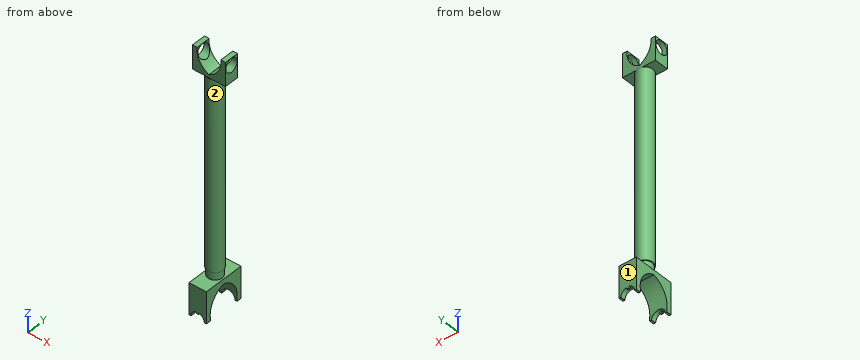
Autodesk Inventor part; units mm, degrees
ref_plane "YZ Plane" through (0, 0, 0) normal (1, 0, 0) x (0, 1, 0)
ref_plane "XZ Plane" through (0, 0, 0) normal (0, 1, 0) x (-1, 0, 0)
ref_plane "XY Plane" through (0, 0, 0) normal (0, 0, 1) x (1, 0, 0)
sketch "Sketch1" plane through (0, 0, 0) normal (0, 0, 1) x (1, 0, 0)
  circle A0 centre (0, 0) radius 5
  dimension "d0" = 10
extrude "Extrusion1" add sketch "Sketch1" against normal blind 120
sketch "Sketch2" plane through (0, 0, -120) normal (0, 0, -1) x (-1, 0, 0)
  circle A0 centre (0, 0) radius 4.5
  dimension "d3" = 9
extrude "Extrusion2" add sketch "Sketch2" along normal blind 5
sketch "Sketch3" plane through (0, 0, 0) normal (0, 0, 1) x (1, 0, 0)
  circle A0 centre (0, 0) radius 5
  line L0 (0, 0) -> (10, 0)
  line L1 (10, 0) -> (-10.5, 0)
  line L2 (0, 0) -> (0, 4.5)
  line L3 (0, 4.5) -> (0, -4.5)
  line L4 (0, -4.5) -> (-10.5, -4.5)
  line L5 (-10.5, -4.5) -> (-10.5, 0)
  line L6 (-10.5, 0) -> (-10.5, 4.5)
  line L7 (-10.5, 4.5) -> (0, 4.5)
  line L8 (0, 4.5) -> (10.5, 4.5)
  line L9 (10.5, 4.5) -> (10.5, -4.5)
  line L10 (10.5, -4.5) -> (0, -4.5)
  dimension "d8" = 4.5
  dimension "d50" = 10.5
  dimension "d52" = 10.5
  dimension "d53" = 4.5
extrude "Extrusion3" add sketch "Sketch3" along normal blind 15 contours L0 L2 L8 A0 | A0 L8 L9 L10 | A0 L10 L3 L0 | L3 L4 A0 L1 | L1 A0 L7 L2 | A0 L1 L6 L7 | L4 L5 L1 A0
sketch "Sketch4" plane through (-10.5, -4.5, 0) normal (0, -1, 0) x (1, 0, 0)
  line L0 (0, 0) -> (8.3206, 0)
  line L1 (12.6794, 0) -> (8.3206, 0)
  line L2 (12.6794, 0) -> (21, 0)
  line L3 (21, 0) -> (21, 15)
  line L4 (0, 15) -> (21, 15)
  line L5 (0, 0) -> (0, 15)
  line L6 (10.5, 0) -> (10.5, 2)
  line L7 (0, 15) -> (21, 15)
  line L8 (0, 15) -> (3, 15)
  line L9 (21, 15) -> (18, 15)
  arc A0 (3, 15) -> (10.5, 2) centre (15.2653, 13.4127) ccw
  line L10 (10.5, 2) -> (10.5, 15)
  line L11 (4.5527, 7.2323) -> (0, 7.2323)
  line L12 (0, 0) -> (0, 15)
  line L13 (4.5527, 7.2323) -> (4.5527, 0)
  line L14 (16.4473, 7.2323) -> (21, 7.2323)
  line L15 (16.4473, 7.2323) -> (16.4473, 0)
  arc A1 (10.5, 2) -> (18, 15) centre (5.7347, 13.4127) ccw
  dimension "d12" = 2
  dimension "d13" = 3
  dimension "d14" = 3
extrude "Extrusion4" cut sketch "Sketch4" against normal blind 15 contours A0 L4 L10 | L10 L4 A1
sketch "Sketch5" plane through (10.5, -4.5, 0) normal (1, 0, 0) x (0, 0, -1)
  line L0 (0, 0) -> (0, 9)
  line L1 (0, 9) -> (-15, 9)
  line L2 (-15, 0) -> (-15, 9)
  line L3 (0, 0) -> (-15, 0)
  line L4 (-15, 0) -> (-15, 9)
  line L5 (-15, 4.5) -> (-10.5, 4.5)
  line L6 (0, 9) -> (0, 0)
  circle A0 centre (-10.5, 4.5) radius 4.25
  point P0 (0, 4.5)
  dimension "d19" = 4.5
  dimension "d20" = 8.5
extrude "Extrusion5" cut sketch "Sketch5" against normal blind 37.25 contours A0
sketch "Sketch6" plane through (0, 0, -125) normal (0, 0, -1) x (-1, 0, 0)
  circle A0 centre (0, 0) radius 4.5
  line L0 (0, 0) -> (0, 13)
  line L1 (0, -4.5) -> (0, 4.5)
  line L2 (0, 13) -> (0, -13)
  line L3 (0, -13) -> (-5.5, -13)
  line L4 (-5.5, -13) -> (5.5, -13)
  line L5 (5.5, -13) -> (5.5, 13)
  line L6 (5.5, 13) -> (-5.5, 13)
  line L7 (-5.5, 13) -> (-5.5, -13)
  dimension "d23" = 13
  dimension "d24" = 26
  dimension "d25" = 5.5
  dimension "d26" = 11
extrude "Extrusion6" add sketch "Sketch6" along normal blind 25
sketch "Sketch7" plane through (5.5, -13, -125) normal (1, 0, 0) x (0, 0, -1)
  line L0 (0, 26) -> (0, 0)
  line L1 (0, 0) -> (25, 0)
  line L2 (25, 26) -> (25, 0)
  line L3 (0, 26) -> (25, 26)
  line L4 (25, 26) -> (25, 0)
  line L5 (25, 26) -> (25, 23)
  line L6 (25, 0) -> (25, 3)
  line L7 (25, 23) -> (18, 23)
  line L8 (0, 8.5) -> (0, 17.5)
  line L9 (0, 13) -> (3, 13)
  arc A0 (18, 23) -> (3, 13) centre (16.2622, 9.3566) ccw
  line L10 (25, 3) -> (18, 3)
  line L11 (18, 3) -> (18, 23)
  arc A1 (3, 13) -> (18, 3) centre (16.3321, 16.7481) ccw
  point P0 (-125, 13)
  dimension "d29" = 3
  dimension "d30" = 3
  dimension "d32" = 7
  dimension "d33" = 3
extrude "Extrusion7" cut sketch "Sketch7" against normal blind 25 contours L2 L10 L11 L7 | A0 L11 A1
sketch "Sketch8" plane through (-5.5, 13, -125) normal (0, 1, 0) x (1, 0, 0)
  line L0 (0, 0) -> (11, 0)
  line L1 (11, 0) -> (11, 25)
  line L2 (0, 25) -> (11, 25)
  line L3 (0, 0) -> (0, 25)
  line L4 (5.5, 25) -> (5.5, 20)
  circle A0 centre (5.5, 20) radius 4.25
  line L5 (1.25, 20) -> (0, 20)
  line L6 (0, 18) -> (0, 25)
  line L7 (9.75, 20) -> (11, 20)
  line L8 (11, 25) -> (11, 18)
  point P0 (5.5, -125)
  dimension "d36" = 5
  dimension "d37" = 8.5
extrude "Extrusion8" cut sketch "Sketch8" against normal blind 30 contours L3 L2 L4 A0 L5 | L7 A0 L4 L2 L1 | A0
sketch "Sketch9" plane through (-5.5, 13, -125) normal (0, 1, 0) x (1, 0, 0)
  line L0 (1.25, 20) -> (0, 20)
  line L1 (0, 0) -> (0, 20)
  line L2 (0, 0) -> (11, 0)
  line L3 (11, 0) -> (11, 20)
  line L4 (11, 20) -> (9.75, 20)
  arc A0 (1.25, 20) -> (9.75, 20) centre (5.5, 20) ccw
  arc A1 (1.25, 20) -> (9.75, 20) centre (5.5, 20) ccw
  line L5 (5.5, 15.75) -> (5, 15.75)
  line L6 (5, 15.75) -> (4.5, 15.75)
  line L7 (4.5, 15.75) -> (6.5, 15.75)
  line L8 (6.5, 15.75) -> (6.1213, 16.7351)
  line L9 (6.1213, 16.7351) -> (5.5, 16.7351)
  line L10 (5.5, 16.7351) -> (5.5, 15.75)
  line L11 (4.5, 15.75) -> (4.8787, 16.7351)
  line L12 (4.8787, 16.7351) -> (5.5, 16.7351)
  line L13 (0, 20) -> (1.25, 20)
  arc A2 (1.25, 20) -> (9.75, 20) centre (5.5, 20) ccw
  line L14 (9.75, 20) -> (11, 20)
  line L15 (11, 0) -> (11, 20)
  line L16 (11, 0) -> (0, 0)
  line L17 (0, 0) -> (0, 20)
  point P0 (5.5, -125)
  point P1 (4.5421, 15.8594)
  point P2 (6.4579, 15.8594)
  dimension "d40" = 0.5
  dimension "d41" = 0.5
  dimension "d42" = 2
extrude "Extrusion9" add sketch "Sketch9" against normal blind 1 contours L11 L12 L10 A0 | L10 L9 L8 A0
sketch "Sketch10" plane through (-5.5, -13, -125) normal (0, -1, 0) x (1, 0, 0)
  line L0 (0, -20) -> (1.25, -20)
  arc A0 (9.75, -20) -> (1.25, -20) centre (5.5, -20) ccw
  line L1 (9.75, -20) -> (11, -20)
  line L2 (11, 0) -> (11, -20)
  line L3 (11, 0) -> (0, 0)
  line L4 (0, 0) -> (0, -20)
  arc A1 (6.4579, -15.8594) -> (4.5421, -15.8594) centre (5.5, -20) ccw
  line L5 (5.5, -15.75) -> (4.5, -15.75)
  line L6 (4.5, -15.75) -> (6.5, -15.75)
  line L7 (6.1213, -16.7351) -> (6.4579, -15.8594)
  line L8 (6.5, -15.75) -> (6.1213, -16.7351)
  line L9 (4.5421, -15.8594) -> (4.8787, -16.7351)
  line L10 (6.1213, -16.7351) -> (4.8787, -16.7351)
  line L11 (4.8787, -16.7351) -> (4.5, -15.75)
  point P0 (5.5, 125)
  dimension "d45" = 1
  dimension "d46" = 2
extrude "Extrusion10" add sketch "Sketch10" against normal blind 1 contours A0 L7 L10 L9
Source: CAD feature listing. Evaluate the final solid. Frame: model axes, mm. Face numbers are marked on the shaded views. Coordinates: 2 decimals unless noted, no trailing zeros. Loops run counter-clockwise (first coordinate to the right, second up) from the corner with the lowest first, then second, coordinate; pieces in that order, holes last. Notation, with made-up numbers: (2, -21) -> (59, -21) arc R21 ccw to (59, 5) -> close; hole circle Ø3 at (70.5, 25). An arc over 180 degrees is marked (long way). Answer in a Markdown table with one row per item. Add a question column.
Q1. Contact query for flat-ended pins moving along their axis: pin 1 Ø8 at (x, z) = (-1, -33.5) entering from -Y; pin 2 Ø7.5 at (y, z) = (0, 10.5) entering from -X; pin 3 Ø5 at (y, z) = (0.5, -64) entering from -X; pin 4 Ø0.8 at (x, y) = (0.5, 12.5) entering from -Z. Output: stop coordinate, or through.
Q2. Section C-C on z = -37.5. Return the cut outline in (x, y), and give its area (3 significant figures).
Q3. Ray query, line 1 along Y through (x, z) = (8.9, 10.5); line 2 along Z through (x, y) = (8.95, 0); line 3 along X through (y, z) = (-2.5, -121.5). Return the intervals inside material, ascending.
Q4. Section B-B on y = -2.75. Return the cut outline in (x, z).
Q5. Pull-direction query (Z, two-part tool) for the marked faces 1 and 2; classes: pulls with the +Z half, pulls with the -Z half, needs draft (parallel to the pull), parting line crosses it, or undercut.
Q6. Section A-A on z = 10.5. Return the cut outline in (x, y).
Computed values:
| question | item | result |
|---|---|---|
| 1 | pin 1 | stops at y = -5 |
| 1 | pin 2 | passes through |
| 1 | pin 3 | stops at x = -5 |
| 1 | pin 4 | stops at z = -141.74 |
| 2 | outline | circle Ø10 at (0, 0) |
| 2 | area | 78.5 mm^2 |
| 3 | line 1 | y = -4.5 to -4.25, 4.25 to 4.5 |
| 3 | line 2 | z = 0 to 6.25, 14.75 to 15 |
| 3 | line 3 | x = -3.74 to 3.74 |
| 4 | outline | (-10.5, 0) -> (-4.18, 0) -> (-4.18, -120) -> (-3.56, -120) -> (-3.56, -125) -> (-5.5, -125) -> (-5.5, -129.1) -> (5.5, -129.1) -> (5.5, -125) -> (3.56, -125) -> (3.56, -120) -> (4.18, -120) -> (4.18, 0) -> (10.5, 0) -> (10.5, 7.26) -> (5.96, 7.26) arc R12.37 cw to (0, 2) arc R12.37 cw to (-5.96, 7.26) -> (-10.5, 7.26) -> close; (-10.5, 13.74) -> (-7.6, 13.74) arc R12.37 cw to (-7.5, 15) -> (-10.5, 15) -> close; (7.5, 15) arc R12.37 cw to (7.6, 13.74) -> (10.5, 13.74) -> (10.5, 15) -> close |
| 5 | face 1 | needs draft |
| 5 | face 2 | undercut |
| 6 | outline | (-10.5, -4.5) -> (-7.25, -4.5) -> (-7.25, -4.25) -> (-10.5, -4.25) -> close; (-10.5, 4.25) -> (-7.25, 4.25) -> (-7.25, 4.5) -> (-10.5, 4.5) -> close; (7.25, -4.5) -> (10.5, -4.5) -> (10.5, -4.25) -> (7.25, -4.25) -> close; (7.25, 4.25) -> (10.5, 4.25) -> (10.5, 4.5) -> (7.25, 4.5) -> close |
